Here's how the part is built. I have some questions about the finished solid (model axes, mm). A direction names the side the tool comes from. Give positions to 0.01 mm unless a question says otherwise; leave off trailing zeros. Loops run counter-clockwise (first coordinate to the right, second up) from the corner with the lowest first, then second, coordinate; pieces in that order, holes last. Notation, with made-up numbers: (26, 23) -> (61, 23) arc R15 ccw to (61, 49) -> close; hole circle Ø4 at (-28.75, 45.5). An arc over 180 degrees is marked (long way). Answer in a Markdown table with one row per item. Add a question column.
Item 1: If we section it at B-B (x = 0): Write out the boundary of the cut face in (y, z), then the cut area to 3 significant figures.
Item 2: Which directions (+Z, -Z, +X, -X, +Y, -Y) give clear straight access to the entire face, cutting with the end or side of a thin tool? Please do faces 4 (the face through (-5.2, 0, -0.1)), 5 (the face through (3, 2, -6)).
Item 3: If we section it at A-A (z = 0): Write out the boundary of the cut face in (x, y), then the cut area to 3 significant figures.
Item 4: We'd pull the mould along X, two halves only. Please class faces 1 (the face through (-4.9, 8, 1.6)), 2 (the face through (-4.88, 4.06, -1.08)), 3 (the face through (-7.81, 0.49, -1.73)): released by +X, released by -X, zero draft, split by the parting line, or undercut.
Item 5: If I drill on line 1 (X direction, y = 5.75, z = 0); line 2 (Y direction, x = 2.25, z = 6.5); line 3 (X direction, y = 5.25, z = -2.5), over which ranges is the centre line in solid material (lowest first)?
Item 6: If we section it at D-D (y = 1.25): Write out the boundary of the cut face in (x, z).
Item 7: If we section it at C-C (y = 4): Write out the boundary of the cut face in (x, z).
Item 8: For P1, Ø2, axis at x = -1.5, z = -3.5, coming from the -Y side; P2, Ø1, axis at x = -6, y = 5, coming from the +Z side; P3, Ø1.5, axis at x = -2, y = 3.5, coming from the -Z side; P4, Ø2, axis at x = 2.5, y = 4, coming from the +Z side, each with a flat end and sliding along its axis, tell me the tip position at first contact or that it passes through.
```python
from build123d import *

# Parameters (mm, degrees)
SKETCH1_R           = 8
BOSS_EXTRUDE1_DEPTH = 2
SKETCH2_R           = 6.5
BOSS_EXTRUDE2_DEPTH = 6
SKETCH3_R           = 5
CUT_EXTRUDE1_DEPTH  = 8
CHAMFER1_SIZE       = 1
CHAMFER2_SIZE       = 1
CHAMFER2_SIZE2      = 0.087488664


with BuildPart() as part:
    # Sketch1 → Boss-Extrude1 (new body)
    with BuildSketch(Plane(origin=(0, 0, 0), x_dir=(1, 0, 0), z_dir=(0, 1, 0))):
        with Locations(Location((0, 0, 0), (0, 0, 270))):
            Circle(SKETCH1_R)
    extrude(amount=BOSS_EXTRUDE1_DEPTH)

    # Sketch2 → Boss-Extrude2 (add)
    with BuildSketch(Plane(origin=(0, 2, 0), x_dir=(1, 0, 0), z_dir=(0, 1, 0))):
        with Locations(Location((0, 0, 0), (0, 0, 270))):
            Circle(SKETCH2_R)
    extrude(amount=BOSS_EXTRUDE2_DEPTH)

    # Sketch3 → Cut-Extrude1 (cut)
    with BuildSketch(Plane(origin=(0, 8, 0), x_dir=(1, 0, 0), z_dir=(0, 1, 0))):
        with Locations(Location((0, 0, 0), (0, 0, 270))):
            Circle(SKETCH3_R)
    extrude(amount=-CUT_EXTRUDE1_DEPTH, mode=Mode.SUBTRACT)

    # Chamfer1
    chamfer1_edges = [part.edges().sort_by_distance(p)[0] for p in [
        (0, 8, -6.5),
    ]]
    chamfer(chamfer1_edges, length=CHAMFER1_SIZE)

    # Chamfer2
    chamfer2_edges = [part.edges().sort_by_distance(p)[0] for p in [
        (0, 2, -8),
    ]]
    chamfer2_side = [part.faces().sort_by_distance(p)[0] for p in [
        (0, 1, -8),
    ]]
    chamfer(chamfer2_edges, length=CHAMFER2_SIZE, length2=CHAMFER2_SIZE2, reference=chamfer2_side[0])


solid = part.part
```
Recorded:
| question | item | result |
|---|---|---|
| 1 | outline | (0, -8) -> (1, -8) -> (2, -7.91) -> (2, -6.5) -> (7, -6.5) -> (8, -5.5) -> (8, -5) -> (0, -5) -> close; (0, 5) -> (8, 5) -> (8, 5.5) -> (7, 6.5) -> (2, 6.5) -> (2, 7.91) -> (1, 8) -> (0, 8) -> close |
| 1 | area | 28.9 mm^2 |
| 2 | face 4 | +Z, -Z, +X, -X, -Y |
| 2 | face 5 | +Y |
| 3 | outline | (-8, 0) -> (-5, 0) -> (-5, 8) -> (-5.5, 8) -> (-6.5, 7) -> (-6.5, 2) -> (-7.91, 2) -> (-8, 1) -> close; (5, 0) -> (8, 0) -> (8, 1) -> (7.91, 2) -> (6.5, 2) -> (6.5, 7) -> (5.5, 8) -> (5, 8) -> close |
| 3 | area | 28.9 mm^2 |
| 4 | face 1 | zero draft |
| 4 | face 2 | undercut |
| 4 | face 3 | split by the parting line |
| 5 | line 1 | x = -6.5 to -5, 5 to 6.5 |
| 5 | line 2 | y = 0 to 2 |
| 5 | line 3 | x = -6 to -4.33, 4.33 to 6 |
| 6 | outline | circle Ø15.96 at (0, 0); hole circle Ø10 at (0, 0) |
| 7 | outline | circle Ø13 at (0, 0); hole circle Ø10 at (0, 0) |
| 8 | P1 | passes through |
| 8 | P2 | stops at z = 3.46 |
| 8 | P3 | stops at z = -6.38 |
| 8 | P4 | stops at z = 6.32 |
